from build123d import *

# Parameters (mm, degrees)
SKETCH_1_R               = 65
SKETCH_1_R_2             = 60
EXTRUDE_1_DEPTH          = 300
SKETCH_2_R               = 85
SKETCH_2_R_2             = 65
EXTRUDE_1_2_DEPTH        = 8
SKETCH_3_R               = 2
CUT_EXTRUDE_1_DEPTH      = 301
SKETCH_4_R               = 85
SKETCH_4_R_2             = 65
EXTRUDE_2_DEPTH          = 8
SKETCH_5_R               = 2
CUT_EXTRUDE_2_DEPTH      = 1
CUT_EXTRUDE_2_DEPTH_BACK = 301


with BuildPart() as part:
    # 草图1 → Extrude 1 (new body)
    with BuildSketch(Plane(origin=(0, 0, 0), x_dir=(1, 0, 0), z_dir=(0, 1, 0))):
        Circle(SKETCH_1_R)
        Circle(SKETCH_1_R_2, mode=Mode.SUBTRACT)
    extrude(amount=EXTRUDE_1_DEPTH)

    # 草图2 → Extrude 1 2 (add)
    with BuildSketch(Plane(origin=(0, 300, 0), x_dir=(1, 0, 0), z_dir=(0, 1, 0))):
        Circle(SKETCH_2_R)
        Circle(SKETCH_2_R_2, mode=Mode.SUBTRACT)
    extrude(amount=-EXTRUDE_1_2_DEPTH)

    # 草图3 → 切除-拉伸1 (cut, through all)
    with BuildSketch(Plane(origin=(0, 300, 0), x_dir=(1, 0, 0), z_dir=(0, 1, 0))):
        with Locations((0, 75)):
            Circle(SKETCH_3_R)
        with Locations((64.951905284, 37.5)):
            Circle(SKETCH_3_R)
        with Locations((64.951905284, -37.5)):
            Circle(SKETCH_3_R)
        with Locations((0, -75)):
            Circle(SKETCH_3_R)
        with Locations((-64.951905284, -37.5)):
            Circle(SKETCH_3_R)
        with Locations((-64.951905284, 37.5)):
            Circle(SKETCH_3_R)
    extrude(amount=-CUT_EXTRUDE_1_DEPTH, mode=Mode.SUBTRACT)

    # 草图4 → 凸台-拉伸2 (add)
    with BuildSketch(Plane.XZ):
        Circle(SKETCH_4_R)
        Circle(SKETCH_4_R_2, mode=Mode.SUBTRACT)
    extrude(amount=-EXTRUDE_2_DEPTH)

    # 草图5 → 切除-拉伸2 (cut, two sides)
    with BuildSketch(Plane.XZ) as cut_extrude_2_sk:
        with Locations((0, 75)):
            Circle(SKETCH_5_R)
        with Locations((64.951905284, 37.5)):
            Circle(SKETCH_5_R)
        with Locations((64.951905284, -37.5)):
            Circle(SKETCH_5_R)
        with Locations((0, -75)):
            Circle(SKETCH_5_R)
        with Locations((-64.951905284, -37.5)):
            Circle(SKETCH_5_R)
        with Locations((-64.951905284, 37.5)):
            Circle(SKETCH_5_R)
    extrude(amount=CUT_EXTRUDE_2_DEPTH, mode=Mode.SUBTRACT)
    extrude(cut_extrude_2_sk.sketch, amount=-CUT_EXTRUDE_2_DEPTH_BACK, mode=Mode.SUBTRACT)


solid = part.part
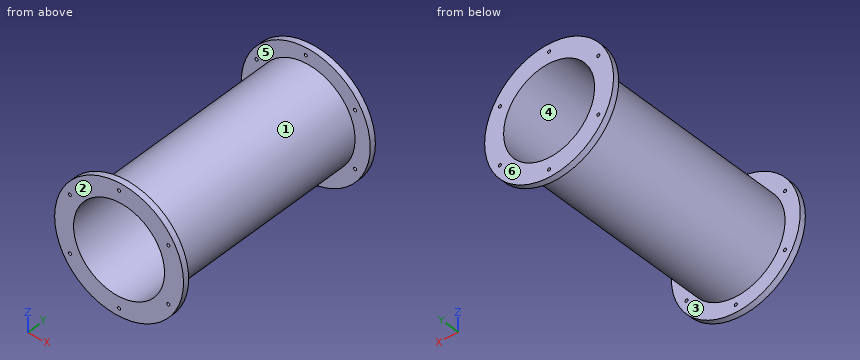
Geometry check sheet. Reference: the model listing, model coordinates, mm. Face numbers are marked on the shaded views. A direction names the side the tool comes from. Round coordinates to 2 decimals unless told otherwise and drop trailing zeros. Loops run counter-clockwise (first coordinate to the right, second up) from the corner with the lowest first, then second, coordinate; pieces in that order, holes last.
Item 1: Gauge pin test, flat ends, axial feed: pin 1 (10 mm diameter, centred on y = 269.5, z = -37.5, fed in from -X); pin 2 (6.5 mm diameter, centred on x = 64.95, z = 37.5, fed in from -Y); pin 3 (3.5 mm diameter, centred on x = -64.95, z = 37.5, fed in from +Y); pin 4 (1 mm diameter, centred on y = 200.5, z = 45, fed in from -X). Record the tip position at first contact, or that the pin passes through.
Item 2: Thickness scan on line 1 (X direction, y = 167, z = 1.5); line 2 (Y direction, x = -77, z = -28.5); line 3 (X direction, y = 298, z = 37). Record the ranges inside material, lowest first.
Item 3: Mould release check, pull along Y, two halves, no side actions. Record for the marked faces 3, 4, 5 and 6: pulls with the +Y half, pulls with the -Y half, needs draft (parallel to the pull), parting line crosses it, or undercut.
Item 4: Cross-section at A-A on x = -25.5. Record the boundary of the cut face in (y, z).
Item 5: Cross-section at B-B on z = -14. Record the boundary of the cut face in (x, y), then the cut area to 3 significant figures.
Item 6: Cross-section at C-C on y = 255. Record the boundary of the cut face in (x, z).
Item 7: Access from +Z, -Z, +X, -X, +Y, -Y to the whole of each face (thin tool, end or side, straight path). Record for the marked faces 1 and 2.
Answer sheet:
1. pin 1: stops at x = -56.29
1. pin 2: stops at y = 0
1. pin 3: passes through
1. pin 4: stops at x = -47.38
2. line 1: x = -64.98 to -59.98, 59.98 to 64.98
2. line 2: y = 0 to 8, 292 to 300
2. line 3: x = -76.52 to -66.89, -63.02 to -47.23, 47.23 to 63.02, 66.89 to 76.52
3. face 3: undercut
3. face 4: needs draft
3. face 5: undercut
3. face 6: pulls with the +Y half
4. outline: (0, -81.08) - (8, -81.08) - (8, -59.79) - (292, -59.79) - (292, -81.08) - (300, -81.08) - (300, -54.31) - (0, -54.31) - close; (0, 54.31) - (300, 54.31) - (300, 81.08) - (292, 81.08) - (292, 59.79) - (8, 59.79) - (8, 81.08) - (0, 81.08) - close
5. outline: (-83.84, 0) - (-58.34, 0) - (-58.34, 300) - (-83.84, 300) - (-83.84, 292) - (-63.47, 292) - (-63.47, 8) - (-83.84, 8) - close; (58.34, 0) - (83.84, 0) - (83.84, 8) - (63.47, 8) - (63.47, 292) - (83.84, 292) - (83.84, 300) - (58.34, 300) - close
5. area: 3,730 mm2
6. outline: circle Ø130 at (0, 0); hole circle Ø120 at (0, 0)
7. face 1: none
7. face 2: +Z, -Z, +X, -X, -Y
